CAD build for the part. Positions are in the model's coordinates, mm. A direction names the side the tool comes from. Coordinates: 2 decimals unless noted, no trailing zeros. Loops run counter-clockwise (first coordinate to the right, second up) from the corner with the lowest first, then second, coordinate; pieces in that order, holes last. Notation, with made-up numbers: (-38.5, 52.5) - (-34.5, 52.5) arc R14 ccw to (-34.5, 77.5) - close; hole circle Ø3 at (53, -22.75). An arc over 180 degrees is marked (long way). Put each result on its own line as item: value.
```python
from build123d import *

# Parameters (mm, degrees)
TOP_PLATE_DEPTH               = 3
SK_TABBLOCKS_W                = 12
SK_TABBLOCKS_H                = 12
TAB_BLOCKS_DEPTH              = 12
SK_SKIRT_W                    = 127.3
SK_SKIRT_H                    = 50.3
SK_SKIRT_W_2                  = 123.2
SK_SKIRT_H_2                  = 46.2
LOCATING_SKIRT_DEPTH          = 9
M3_CLEARANCE_HOLES_DEPTH      = 163.531227769
M3_CLEARANCE_HOLES_DEPTH_BACK = 163.531227769
SK_TABHOLES_R                 = 1.7
SK_VENTS_R                    = 2.1
VENT_HOLES_DEPTH              = 3


with BuildPart() as part:
    # Sk_Plate → Top Plate (new body)
    with BuildSketch(Plane(origin=(0, 52, 0), x_dir=(1, 0, 0), z_dir=(0, 1, 0))):
        with BuildLine():
            Line((4, 0), (128.8, 0))
            ThreePointArc((128.8, 0), (131.628427125, 1.171572875), (132.8, 4))
            Line((132.8, 4), (132.8, 51.8))
            ThreePointArc((132.8, 51.8), (131.628427125, 54.628427125), (128.8, 55.8))
            Line((128.8, 55.8), (4, 55.8))
            ThreePointArc((4, 55.8), (1.171572875, 54.628427125), (0, 51.8))
            Line((0, 51.8), (0, 4))
            ThreePointArc((0, 4), (1.171572875, 1.171572875), (4, 0))
        make_face()
    extrude(amount=TOP_PLATE_DEPTH)

    # Sk_TabBlocks → Tab Blocks (add)
    with BuildSketch(Plane(origin=(0, 43, 0), x_dir=(1, 0, 0), z_dir=(0, 1, 0))):
        with Locations((-3.6, 12)):
            Rectangle(SK_TABBLOCKS_W, SK_TABBLOCKS_H)
        with Locations((136.4, 12)):
            Rectangle(SK_TABBLOCKS_W, SK_TABBLOCKS_H)
        with Locations((-3.6, 43.8)):
            Rectangle(SK_TABBLOCKS_W, SK_TABBLOCKS_H)
        with Locations((136.4, 43.8)):
            Rectangle(SK_TABBLOCKS_W, SK_TABBLOCKS_H)
    extrude(amount=TAB_BLOCKS_DEPTH)

    # Sk_Skirt → Locating Skirt (add)
    with BuildSketch(Plane(origin=(0, 43, 0), x_dir=(1, 0, 0), z_dir=(0, 1, 0))):
        with Locations((66.4, 27.9)):
            Rectangle(SK_SKIRT_W, SK_SKIRT_H)
        with Locations((66.75, 28.25)):
            Rectangle(SK_SKIRT_W_2, SK_SKIRT_H_2, mode=Mode.SUBTRACT)
    extrude(amount=LOCATING_SKIRT_DEPTH)

    # Sk_TabHoles → M3 Clearance Holes (cut, two sides: drawn at the far end of the back side and taken through both)
    with BuildSketch(Plane(origin=(0, 0, 0), x_dir=(1, 0, 0), z_dir=(0, 1, 0)).offset(-M3_CLEARANCE_HOLES_DEPTH_BACK)):
        with Locations(Location((-3.6, 12, 0), (0, 0, 90))):
            Circle(SK_TABHOLES_R)
        with Locations(Location((-3.6, 43.8, 0), (0, 0, 90))):
            Circle(SK_TABHOLES_R)
        with Locations(Location((136.4, 12, 0), (0, 0, 90))):
            Circle(SK_TABHOLES_R)
        with Locations(Location((136.4, 43.8, 0), (0, 0, 90))):
            Circle(SK_TABHOLES_R)
    extrude(amount=M3_CLEARANCE_HOLES_DEPTH + M3_CLEARANCE_HOLES_DEPTH_BACK, mode=Mode.SUBTRACT)

    # Sk_Vents → Vent Holes (cut)
    with BuildSketch(Plane(origin=(0, 52, 0), x_dir=(1, 0, 0), z_dir=(0, 1, 0))):
        with Locations(Location((18, 10, 0), (0, 0, 270))):
            Circle(SK_VENTS_R)
        with Locations(Location((18, 17, 0), (0, 0, 270))):
            Circle(SK_VENTS_R)
        with Locations(Location((18, 24, 0), (0, 0, 270))):
            Circle(SK_VENTS_R)
        with Locations(Location((18, 31, 0), (0, 0, 270))):
            Circle(SK_VENTS_R)
        with Locations(Location((18, 38, 0), (0, 0, 270))):
            Circle(SK_VENTS_R)
        with Locations(Location((18, 45, 0), (0, 0, 270))):
            Circle(SK_VENTS_R)
        with Locations(Location((37, 10, 0), (0, 0, 270))):
            Circle(SK_VENTS_R)
        with Locations(Location((37, 17, 0), (0, 0, 270))):
            Circle(SK_VENTS_R)
        with Locations(Location((37, 24, 0), (0, 0, 270))):
            Circle(SK_VENTS_R)
        with Locations(Location((37, 31, 0), (0, 0, 270))):
            Circle(SK_VENTS_R)
        with Locations(Location((37, 38, 0), (0, 0, 270))):
            Circle(SK_VENTS_R)
        with Locations(Location((37, 45, 0), (0, 0, 270))):
            Circle(SK_VENTS_R)
        with Locations(Location((56, 10, 0), (0, 0, 270))):
            Circle(SK_VENTS_R)
        with Locations(Location((56, 17, 0), (0, 0, 270))):
            Circle(SK_VENTS_R)
        with Locations(Location((56, 24, 0), (0, 0, 270))):
            Circle(SK_VENTS_R)
        with Locations(Location((56, 38, 0), (0, 0, 270))):
            Circle(SK_VENTS_R)
        with Locations(Location((56, 45, 0), (0, 0, 270))):
            Circle(SK_VENTS_R)
        with Locations(Location((75, 10, 0), (0, 0, 270))):
            Circle(SK_VENTS_R)
        with Locations(Location((75, 17, 0), (0, 0, 270))):
            Circle(SK_VENTS_R)
        with Locations(Location((75, 24, 0), (0, 0, 270))):
            Circle(SK_VENTS_R)
        with Locations(Location((75, 38, 0), (0, 0, 270))):
            Circle(SK_VENTS_R)
        with Locations(Location((75, 45, 0), (0, 0, 270))):
            Circle(SK_VENTS_R)
        with Locations(Location((94, 10, 0), (0, 0, 270))):
            Circle(SK_VENTS_R)
        with Locations(Location((94, 17, 0), (0, 0, 270))):
            Circle(SK_VENTS_R)
        with Locations(Location((94, 24, 0), (0, 0, 270))):
            Circle(SK_VENTS_R)
        with Locations(Location((94, 31, 0), (0, 0, 270))):
            Circle(SK_VENTS_R)
        with Locations(Location((94, 38, 0), (0, 0, 270))):
            Circle(SK_VENTS_R)
        with Locations(Location((94, 45, 0), (0, 0, 270))):
            Circle(SK_VENTS_R)
        with Locations(Location((113, 10, 0), (0, 0, 270))):
            Circle(SK_VENTS_R)
        with Locations(Location((113, 17, 0), (0, 0, 270))):
            Circle(SK_VENTS_R)
        with Locations(Location((113, 24, 0), (0, 0, 270))):
            Circle(SK_VENTS_R)
        with Locations(Location((113, 31, 0), (0, 0, 270))):
            Circle(SK_VENTS_R)
        with Locations(Location((113, 38, 0), (0, 0, 270))):
            Circle(SK_VENTS_R)
        with Locations(Location((113, 45, 0), (0, 0, 270))):
            Circle(SK_VENTS_R)
    extrude(amount=VENT_HOLES_DEPTH, mode=Mode.SUBTRACT)


solid = part.part
```
Q1. Pin check, flat tips, straight feed: pin 1 Ø2.5 at (x, z) = (56, -17) entering from +Y; pin 2 Ø6.5 at (x, z) = (94, -31) entering from -Y; pin 3 Ø1 at (y, z) = (48.5, -35) entering from +X; pin 4 Ø2 at (x, y) = (39.5, 46.5) entering from +Z. Stop position of each tip, or through.
Determined:
pin 1: through
pin 2: y = 52
pin 3: x = 130.05
pin 4: z = -2.75
Q2. Slice it at B-B, the plane x = -3.6. Give the cut face in (y, z).
Determined:
outline: (43, -49.8) - (55, -49.8) - (55, -45.5) - (43, -45.5) - close; (43, -42.1) - (55, -42.1) - (55, -37.8) - (43, -37.8) - close; (43, -18) - (55, -18) - (55, -13.7) - (43, -13.7) - close; (43, -10.3) - (55, -10.3) - (55, -6) - (43, -6) - close
Q3. Wall check: L1, parallel to X at y = 49.5, z = -7; L2, parallel to X at y = 49, z = -26; L3, parallel to Z at x = 114.5, y = 47.75. Give the ranges that are in metal, low to high. Write a range as from..to.
Determined:
L1: -9.6..2.4, 2.75..5.15, 128.35..130.05, 130.4..142.4
L2: 2.75..5.15, 128.35..130.05
L3: -53.05..-51.35, -5.15..-2.75
Q4. Mould opens along Z. For faces 4 (the flat face through (-9.6, 49, -12)), 5 (the cylindrical face through (34.95, 53.48, -10.46)), 6 (the flat face through (66, 47, -2.75)) say: +Z half, -Z half, draft (parallel to the pull), parting line (faces both ways), or undercut.
Determined:
face 4: draft
face 5: undercut
face 6: +Z half
Q5. Tool access for faces 1 (the flat face through (2.75, 47, -28)), 2 (the cylindrical face through (53.95, 53.48, -10.46)), 3 (the flat face through (5.15, 47, -28)): list every direction of +Z, -Z, +X, -X, +Y, -Y with a clear straight run to the whole face (end or side of a thin tool).
Determined:
face 1: +Z, -Z, -Y
face 2: +Y, -Y
face 3: -Y
Q6. Slice it at C-C, the plane x = 51. Give the cut face in (y, z), then the cut area to 3 significant figures.
Determined:
outline: (43, -53.05) - (52, -53.05) - (52, -55.8) - (55, -55.8) - (55, 0) - (52, 0) - (52, -2.75) - (43, -2.75) - (43, -5.15) - (52, -5.15) - (52, -51.35) - (43, -51.35) - close
area: 204 mm2
Q7. Slice it at A-A, the plane y = 47.5. State how many separate pieces and enclosed holes the cut face has, then the cut area to 3 significant figures.
Determined:
separate pieces: 5
enclosed holes: 5
area: 1,250 mm2
